Build history of the part. All positions in model axes, mm. A direction names the side the tool comes from. Give positions to 0.01 mm unless a question says otherwise; leave off trailing zeros. Order: outer loops, then holes, each group sorted by start corner. A loop starts at its lowest first (then second) coordinate and runs counter-clockwise, first axis right, second up. Notation, with made-up numbers: (-30.5, 78.25) - (9.5, 78.25) arc R33 ccw to (9.5, 115.25) - close; hole circle Ø2 at (36, 65). An arc over 180 degrees is marked (long way). Use a Markdown table: item, result. Add a question column.
(1) Which spindle directions (+Z, -Z, +X, -X, +Y, -Y) get a long thin tool onto all of the face, cutting with end or side? Do faces 1 (the face through (14.1, -11.5, 16)), 2 (the face through (0, -17, 3)), 3 (the face through (0, -19, 5.2)). Say none if no direction does.
(2) Flat gauge pins, fed straight in: pin 1 (3 mm diameter, centred on x = -15, y = 10, fed in from -Z); pin 2 (4 mm diameter, centred on x = 22, y = -13.5, fed in from -Z); pin 3 (1.5 mm diameter, centred on y = -10, z = 5, fed in from -X); pin 4 (4.5 mm diameter, centred on x = 15, y = 10, fed in from -Z). Where does each tip first touch, or does it go through?
(3) Slice it at C-C (z = 11.75). Write the cut outline in (x, y) (3 decimals).
(4) Slice it at B-B (y = -10). Write the cut outline in (x, z), then the cut area to 3 significant figures.
(5) Slice it at A-A (x = -15). Write the cut outline in (y, z) (3 decimals), then the cut area to 3 significant figures.
(6) Wall check: line 1 (Y direction, x = 15, z = 15.55) (3 decimals); line 2 (X direction, y = 10, z = 16.5); line 3 (Z direction, x = 25, y = -20). Give the ranges that are in metal, low to high.
(7) Mould opens along Z. For faces 4 (the face through (0, 20.125, 9)), 5 (the face through (2, 25.125, 8)), 6 (the face through (0, 19, 5.2)), 7 (the face through (2, 0, 17)) say: +Z half, -Z half, draft (parallel to the pull), parting line (faces both ways), or undercut.
(8) Slice it at D-D (y = -19.5). Write the cut outline in (x, z), then the cut area to 3 significant figures.
Autodesk Fusion 360 part; units mm, degrees
sketch "Sketch1" plane through (0, 0, 0) normal (0, 0, 1) x (1, 0, 0)
  line L0 (26, 17) -> (-26, 17)
  line L1 (-26, 17) -> (-26, -17)
  line L2 (-26, -17) -> (26, -17)
  line L3 (26, -17) -> (26, 17)
  line L4 (-26, 17) -> (26, -17) construction
  line L5 (26, 20.125) -> (-26, 20.125)
  line L6 (-26, 20.125) -> (-26, -20.125)
  line L7 (-26, -20.125) -> (26, -20.125)
  line L8 (26, -20.125) -> (26, 20.125)
  line L9 (-26, 20.125) -> (26, -20.125) construction
  line L10 (26, -20.125) -> (31, -20.125)
  line L11 (31, -20.125) -> (31, 0)
  line L12 (1.75, 0) -> (22.5, 0)
  line L13 (31, 20.125) -> (31, 0)
  line L14 (26, 20.125) -> (31, 20.125)
  line L15 (-26, -20.125) -> (-26, -25.125)
  line L16 (-26, -25.125) -> (31, -25.125)
  line L17 (31, -25.125) -> (31, -20.125)
  line L18 (-26, 25.125) -> (31, 25.125)
  line L19 (31, 25.125) -> (31, 20.125)
  line L20 (-26, 20.125) -> (-26, 25.125)
  dimension "d1" = 52
  dimension "d2" = 34
  dimension "d3" = 52
  dimension "d4" = 40.25
  dimension "d7" = 5
extrude "Extrude1" add sketch "Sketch1" along normal blind 5.2 contours L3 L8 L10 L11 L13 L14 | L0 L5 L6 L8 | L2 L6 L7 L8 | L5 L14 L18 L19 L20 | L7 L10 L15 L16 L17
extrude "Extrude2" add sketch "Sketch1" along normal blind 14 contours L3 L8 L10 L11 L13 L14 | L5 L14 L18 L19 L20 | L7 L10 L15 L16 L17
extrude "Extrude3" add sketch "Sketch1" along normal blind 17 and the other way blind -14
sketch "Sketch2" plane through (0, 0, 17) normal (0, 0, 1) x (-1, 0, 0)
  line L0 (26, -25.125) -> (26, 25.125)
  line L1 (26, 25.125) -> (-31, 25.125)
  line L2 (-31, 25.125) -> (-31, -25.125)
  line L3 (-31, -25.125) -> (26, -25.125)
  circle A0 centre (15, 10) radius 1.75
  circle A1 centre (-15, 10) radius 1.75
  line L4 (-1.75, 0) -> (-22.5, 0)
  circle A2 centre (-15, -10) radius 1.75
  circle A3 centre (15, -10) radius 1.75
  dimension "d14" = 3.5
  dimension "d15" = 3.5
extrude "Extrude4" cut sketch "Sketch2" against normal blind 5 contours A0 | A1 | A2 | A3
chamfer "Chamfer1" distance 1 angle 45 4 edges at (-13.3684, 10.6328, 14) (-13.3684, -9.3672, 14) (16.6316, 10.6328, 14) (16.6316, -9.3672, 14)
chamfer "Chamfer2" distance 1 angle 45 2 edges at (-26, 17, 2.6) (-26, -17, 2.6)
chamfer "Chamfer3" distance 1 angle 45 2 edges at (-26, 19.0625, 5.2) (-26, -19.0625, 5.2)
Solution:
| question | item | result |
|---|---|---|
| 1 | face 1 | +Z, -Z |
| 1 | face 2 | -Z, -X |
| 1 | face 3 | -X |
| 2 | pin 1 | through |
| 2 | pin 2 | z = 14 |
| 2 | pin 3 | x = 26 |
| 2 | pin 4 | z = 14.5 |
| 3 | outline | (-26, -25.125) - (31, -25.125) - (31, 25.125) - (-26, 25.125) - (-26, 20.125) - (26, 20.125) - (26, -20.125) - (-26, -20.125) - close |
| 4 | outline | (-26, 14) - (-17.75, 14) - (-16.75, 15) - (-16.75, 17) - (-26, 17) - close; (-13.25, 15) - (-12.25, 14) - (12.25, 14) - (13.25, 15) - (13.25, 17) - (-13.25, 17) - close; (16.75, 15) - (17.75, 14) - (26, 14) - (26, 0) - (31, 0) - (31, 17) - (16.75, 17) - close |
| 4 | area | 218 mm2 |
| 5 | outline | (-25.125, 0) - (-17, 0) - (-17, 5.2) - (-20.125, 5.2) - (-20.125, 14) - (-12.75, 14) - (-11.75, 15) - (-11.75, 17) - (-25.125, 17) - close; (-8.25, 15) - (-7.25, 14) - (7.25, 14) - (8.25, 15) - (8.25, 17) - (-8.25, 17) - close; (11.75, 15) - (12.75, 14) - (20.125, 14) - (20.125, 5.2) - (17, 5.2) - (17, 0) - (25.125, 0) - (25.125, 17) - (11.75, 17) - close |
| 5 | area | 300 mm2 |
| 6 | line 1 | -25.125 to -11.75, -8.25 to 8.25, 11.75 to 25.125 |
| 6 | line 2 | -26 to -16.75, -13.25 to 13.25, 16.75 to 31 |
| 6 | line 3 | 0 to 5.2, 14 to 17 |
| 7 | face 4 | undercut |
| 7 | face 5 | draft |
| 7 | face 6 | undercut |
| 7 | face 7 | +Z half |
| 8 | outline | (-26, 0) - (31, 0) - (31, 17) - (-26, 17) - (-26, 14) - (26, 14) - (26, 5.2) - (-25, 5.2) - (-26, 4.2) - close |
| 8 | area | 511 mm2 |
